Study the drawing (mm; zero at the part's minimum x, y, z) and answer. A direction names the side the tool comes from. Round coordinates to 2 decimals unless told otherwise and drop trailing zeros. Write each loop counter-clockwise with the first axis right and the second up, starting at its lowest first coordinate (ties: lowest second). Pieces come first, ordered by that corner, then holes. Notation, with made-up numbers: (-37, -15) -> (-8, -15) arc R17 cw to (-8, 9) -> close; hole circle Ø10 at (-39.5, 29). An arc over 180 degrees is marked (long way). One line per question, with ' | ' between items. Start each with the question number.
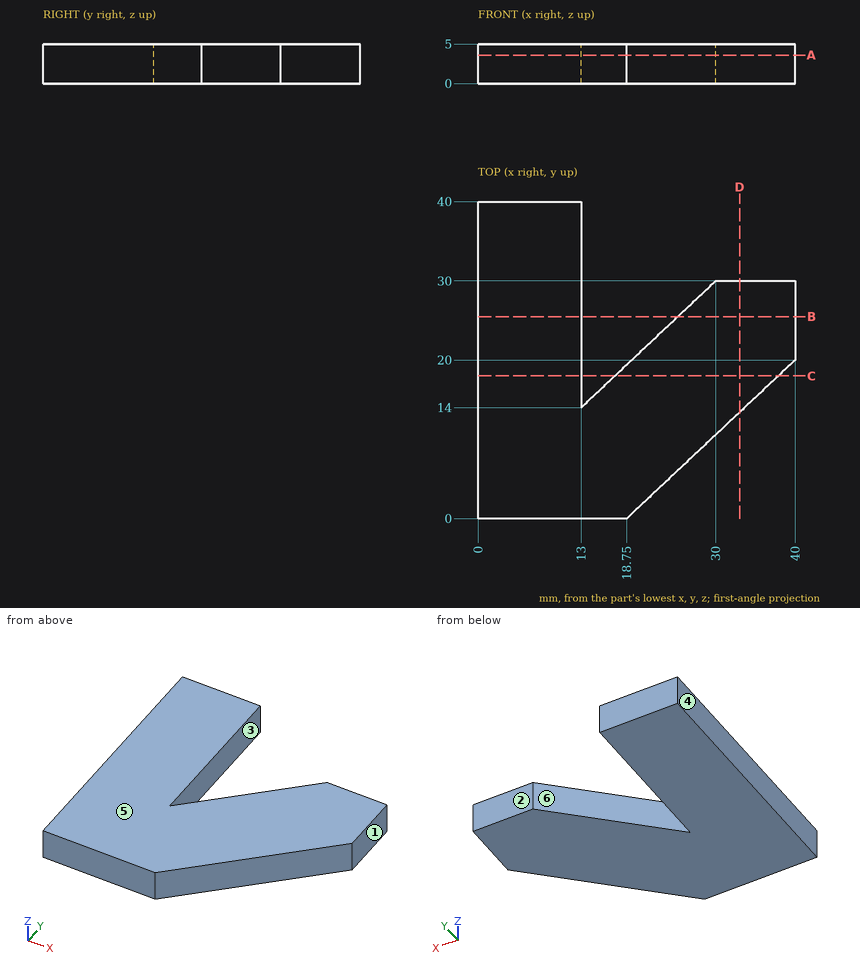
(1) A cutting plane is placed at C-C, the plane y = 18. Determine the outline of the cut face in (x, z) (3 decimals), then the cut area to 3 significant figures.
(2) A cutting plane is placed at A-A, the plane z = 3.6. Determine the outline of the cut face in (x, y), then the cut area to 4 significant figures.
(3) Consider L1, parallel to X at y = 18.5, z = 0.55; L2, parallel to X at y = 25.5, z = 2.5; L3, parallel to X at y = 35, z = 1.45. Determine where each line is inside the solid, lowest interval first.
(4) A cutting plane is placed at B-B, the plane y = 25.5. Determine the outline of the cut face in (x, z).
(5) A cutting plane is placed at D-D, the plane x = 33. Determine the outline of the cut face in (y, z), then the cut area to 3 significant figures.
(6) The mould has two halves that part along X. Classify the marked faces 4, 5 and 6: +X half, -X half, draft (parallel to the pull), parting line (faces both ways), or undercut.
(7) Given pin 1 Ø1.5 at (y, z) = (14, 2.5) entering from +X; pin 2 Ø1.5 at (x, z) = (24, 3.5) entering from +Y; pin 3 Ø2.5 at (x, z) = (34, 2) entering from +Y, each flat-ended and moving along its own axis, determine where each tip first touches the part or whether it passes through.
(8) For the marked faces 1, 2 and 3, determine the directions among +Z, -Z, +X, -X, +Y, -Y from which every point of the face is accessible in a straight line to the end or side of a thin tool.
Returned:
1) outline: (0, 0) -> (13, 0) -> (13, 5) -> (0, 5) -> close; (17.25, 0) -> (37.875, 0) -> (37.875, 5) -> (17.25, 5) -> close | area: 168 mm2
2) outline: (0, 0) -> (18.75, 0) -> (40, 20) -> (40, 30) -> (30, 30) -> (13, 14) -> (13, 40) -> (0, 40) -> close | area: 981.5 mm2
3) L1: 0 to 13, 17.78 to 38.41 | L2: 0 to 13, 25.22 to 40 | L3: 0 to 13
4) outline: (0, 0) -> (13, 0) -> (13, 5) -> (0, 5) -> close; (25.22, 0) -> (40, 0) -> (40, 5) -> (25.22, 5) -> close
5) outline: (13.41, 0) -> (30, 0) -> (30, 5) -> (13.41, 5) -> close | area: 82.9 mm2
6) face 4: -X half | face 5: draft | face 6: undercut
7) pin 1: x = 34.42 | pin 2: y = 25.06 | pin 3: y = 30
8) face 1: +Z, -Z, +X, +Y, -Y | face 2: +Z, -Z, +X, +Y | face 3: +Z, -Z, +Y
